Part model, mm, in its own coordinate system. Coordinates: 2 decimals unless noted, no trailing zeros. Loops run counter-clockwise (first coordinate to the right, second up) from the corner with the lowest first, then second, coordinate; pieces in that order, holes last. Notation, with made-up numbers: (-19, 24.5) - (-7, 24.5) arc R27 ccw to (-7, 53.5) - close; hole circle Ø9 at (-7, -22). An arc over 180 degrees is marked (long way). Use a Markdown table: item, result. Add a question column.
1. Band-saw the part on B-B, the plane y = 0. Give the cut face in (x, z).
2. Band-saw the part on A-A, the plane x = 6. Give the cut face in (y, z), plus the area to 3 significant figures.
3. Band-saw the part on D-D, the plane y = 7. Give the cut face in (x, z), plus the area to 3 significant figures.
4. Band-saw the part on C-C, the plane z = 0.25. Give the cut face in (x, y).
5. Drop flat-ended pins along their axis: pin 1 (1.5 mm diameter, centred on x = -3, y = -5, fed in from -Z); pin 2 (1.2 mm diameter, centred on x = -6, y = 0, fed in from +Z). Give the stop position or say it passes through.
6. Wall check: probe 1 along Y at (x, z) = (6, 0.85); probe 2 along X at (y, z) = (0.5, 0.2); probe 3 along X at (y, z) = (6.25, 1.3). Give the ranges that are in metal, low to high. Write a range as [from, to].
7. Pull direction Y, two halves, no side cores. Call faces 1 (the cylindrical face through (5.2, -0.6, 0.8)), 2 (the flat face through (0, -8, 1)), 3 (the flat face through (-7.6, 0, 1)): pulls with the +Y half, pulls with the -Y half, needs draft (parallel to the pull), parting line crosses it, or undercut.
from build123d import *

# Parameters (mm, degrees)
ESQUISSE1_W        = 15.2
ESQUISSE1_H        = 16
ESQUISSE1_R        = 1
BOSS_EXTRU_1_DEPTH = 1.7
CHANFREIN1_SIZE    = 2.5


with BuildPart() as part:
    # Esquisse1 → Boss.-Extru.1 (new body)
    with BuildSketch(Plane.XY):
        Rectangle(ESQUISSE1_W, ESQUISSE1_H)
        with Locations((-6, 0)):
            Circle(ESQUISSE1_R, mode=Mode.SUBTRACT)
        with Locations((6, 0)):
            Circle(ESQUISSE1_R, mode=Mode.SUBTRACT)
    extrude(amount=BOSS_EXTRU_1_DEPTH)

    # Chanfrein1
    chanfrein1_edges = [part.edges().sort_by_distance(p)[0] for p in [
        (-7.6, 8, 0.85),
        (7.6, 8, 0.85),
        (7.6, -8, 0.85),
        (-7.6, -8, 0.85),
    ]]
    chamfer(chanfrein1_edges, length=CHANFREIN1_SIZE)


solid = part.part
Geometry check:
| question | item | result |
|---|---|---|
| 1 | outline | (-7.6, 0) - (-7, 0) - (-7, 1.7) - (-7.6, 1.7) - close; (-5, 0) - (5, 0) - (5, 1.7) - (-5, 1.7) - close; (7, 0) - (7.6, 0) - (7.6, 1.7) - (7, 1.7) - close |
| 2 | outline | (-7.1, 0) - (-1, 0) - (-1, 1.7) - (-7.1, 1.7) - close; (1, 0) - (7.1, 0) - (7.1, 1.7) - (1, 1.7) - close |
| 2 | area | 20.7 mm^2 |
| 3 | outline | (-6.1, 0) - (6.1, 0) - (6.1, 1.7) - (-6.1, 1.7) - close |
| 3 | area | 20.7 mm^2 |
| 4 | outline | (-7.6, -5.5) - (-5.1, -8) - (5.1, -8) - (7.6, -5.5) - (7.6, 5.5) - (5.1, 8) - (-5.1, 8) - (-7.6, 5.5) - close; hole circle Ø2 at (-6, 0); hole circle Ø2 at (6, 0) |
| 5 | pin 1 | stops at z = 0 |
| 5 | pin 2 | passes through |
| 6 | probe 1 | y = [-7.1, -1], [1, 7.1] |
| 6 | probe 2 | x = [-7.6, -6.87], [-5.13, 5.13], [6.87, 7.6] |
| 6 | probe 3 | x = [-6.85, 6.85] |
| 7 | face 1 | undercut |
| 7 | face 2 | pulls with the -Y half |
| 7 | face 3 | needs draft |
